The model under review builds one solid part; all positions refer to its coordinate system, in mm. A direction names the side the tool comes from. Round coordinates to 2 decimals unless told otherwise and drop trailing zeros. Write each loop counter-clockwise with the first axis right and the second up, starting at its lowest first coordinate (ties: lowest second). Pieces come first, ordered by that corner, then holes. Notation, with made-up numbers: (59, -24.75) -> (101, -24.75) arc R13 ccw to (101, -20.75) -> close; hole circle Ø8 at (87.25, -2). An arc over 180 degrees is marked (long way). Use CSV: the item, a comma, the result in double quotes. Start each with the question number.
1) Take a section at A-A, the plane y = -3. Give the boundary of the cut face in (x, z), then the cut area to 3 significant figures.
2) Mouldability with a two-part tool opening along Y and no side actions: class faces 1 (the face through (0, 15.5, 0)), 2 (the face through (15.5, 0, 0)), 3 (the face through (0, 0, -12.5)) as released by +Y, released by -Y, zero draft, split by the parting line, or undercut.
3) Wall thickness on probe 1 along X at (y, z) = (12, -1.5): over which ranges is the line inside the solid? List them lowest first. Write a range as [from, to].
4) Machinability: for faces 4 (the face through (0, 0, 15.5)), 5 (the face through (0, 0, 12.5)), which of the approach directions +Z, -Z, +X, -X, +Y, -Y give a long, thin tool a straight path to every point of the face, cutting with its end or side? Answer none if there is none.
from build123d import *

# Parameters (mm, degrees)
F0_W     = 31
F0_H     = 31
F0_W_2   = 25
F0_H_2   = 25
F1_DEPTH = 15.5
F2_W     = 25
F2_H     = 25
F3_DEPTH = 3
F4_W     = 25
F4_H     = 25
F5_DEPTH = 3


with BuildPart() as f1:
    # F0 (on Front) → F1 (new body, symmetric)
    with BuildSketch(Plane.XZ):
        Rectangle(F0_W, F0_H)
        Rectangle(F0_W_2, F0_H_2, mode=Mode.SUBTRACT)
    extrude(amount=F1_DEPTH, both=True)

    # F2 (on face) → F3 (join)
    with BuildSketch(Plane.XZ.offset(15.5)):
        Rectangle(F2_W, F2_H)
    extrude(amount=-F3_DEPTH)

    # F4 (on face) → F5 (join)
    with BuildSketch(Plane(origin=(0, 15.5, 0), x_dir=(-1, 0, 0), z_dir=(0, 1, 0))):
        Rectangle(F4_W, F4_H)
    extrude(amount=-F5_DEPTH)


solid = f1.part
Values found:
1,outline,"(-15.5, -15.5) -> (15.5, -15.5) -> (15.5, 15.5) -> (-15.5, 15.5) -> close; hole (-12.5, -12.5) -> (12.5, -12.5) -> (12.5, 12.5) -> (-12.5, 12.5) -> close"
1,area,"336 mm²"
2,face 1,"released by +Y"
2,face 2,"zero draft"
2,face 3,"undercut"
3,probe 1,"[-15.5, -12.5], [12.5, 15.5]"
4,face 4,"+Z, +X, -X, +Y, -Y"
4,face 5,"none"
